```python
from build123d import *

# Parameters (mm, degrees)
SKETCH2_W           = 34
SKETCH2_H           = 27.6
SKETCH2_R           = 2
BOSS_EXTRUDE1_DEPTH = 4
SKETCH3_W           = 34
SKETCH3_H           = 4
BOSS_EXTRUDE2_DEPTH = 47
FILLET1_R           = 9
SKETCH4_R           = 4.5
CUT_EXTRUDE1_DEPTH  = 5


with BuildPart() as part:
    # Sketch2 → Boss-Extrude1 (new body)
    with BuildSketch(Plane(origin=(0, 0, 0), x_dir=(1, 0, 0), z_dir=(0, 1, 0))):
        Rectangle(SKETCH2_W, SKETCH2_H)
        with Locations((0, -7.8)):
            Circle(SKETCH2_R, mode=Mode.SUBTRACT)
    extrude(amount=BOSS_EXTRUDE1_DEPTH)

    # Sketch3 → Boss-Extrude2 (add)
    with BuildSketch(Plane(origin=(0, 4, 0), x_dir=(1, 0, 0), z_dir=(0, 1, 0))):
        with Locations((0, 11.8)):
            Rectangle(SKETCH3_W, SKETCH3_H)
    extrude(amount=BOSS_EXTRUDE2_DEPTH)

    # Fillet1
    fillet1_edges = [part.edges().sort_by_distance(p)[0] for p in [
        (-17, 51, -11.8),
        (17, 51, -11.8),
    ]]
    fillet(fillet1_edges, radius=FILLET1_R)

    # Sketch4 → Cut-Extrude1 (cut, through all)
    with BuildSketch(Plane.XY.offset(-9.8)):
        with Locations((0, 39)):
            Circle(SKETCH4_R)
    extrude(amount=-CUT_EXTRUDE1_DEPTH, mode=Mode.SUBTRACT)


solid = part.part
```
CAD build for the part. Positions are in the model's coordinates, mm. Round coordinates to 2 decimals unless told otherwise and drop trailing zeros. Loops run counter-clockwise (first coordinate to the right, second up) from the corner with the lowest first, then second, coordinate; pieces in that order, holes last. Notation, with made-up numbers: (72, -22.75) - (114, -22.75) arc R21 cw to (114, -2.75) - close; hole circle Ø2 at (-27, 18). An arc over 180 degrees is marked (long way). Return JSON: item names as keys, results as strings. Group by question number.
Q1. Flat gauge pin, fed straight in: pin 1 Ø5 at (x, y) = (11, 42) entering from +Z. Where does the tip first touch, or does it go through?
Q2. Two-plate mould, pull along Y, no slides. Class faces 1 (the face through (0, 27, -9.8)), 2 (the face through (0, 4, 2)), 3 (the face through (-0.98, 34.61, -11.77)): +Y half, -Y half, draft (parallel to the pull), parting line (faces both ways), or undercut.
Q3. Band-saw the part on B-B on z = -11. Give the cut face in (x, y), plus the area to 3 significant figures.
Q4. Band-saw the part on A-A on z = 7.8. Give the cut face in (x, y).
Q5. Drill centre lines: line 1 along X through (y, z) = (1.4, 7.8); line 2 along Z through (x, y) = (0, 2); line 3 along Y through (x, z) = (0, -10.7). Where is each one in solid material? Low to high. Write a range as [from, to].
Q6. Band-saw the part on D-D on x = 0. Give the cut face in (y, z), plus the area to 3 significant figures.
Q7. Band-saw the part on C-C on y = 39. Give the cut face in (x, z).
Solutions:
{
 "1": {"pin 1": "stops at z = -9.8"},
 "2": {"face 1": "draft", "face 2": "+Y half", "face 3": "undercut"},
 "3": {"outline": "(-17, 0) - (17, 0) - (17, 42) arc R9 ccw to (8, 51) - (-8, 51) arc R9 ccw to (-17, 42) - close; hole circle Ø9 at (0, 39)", "area": "1,640 mm^2"},
 "4": {"outline": "(-17, 0) - (-2, 0) - (-2, 4) - (-17, 4) - close; (2, 0) - (17, 0) - (17, 4) - (2, 4) - close"},
 "5": {"line 1": "x = [-17, -2], [2, 17]", "line 2": "z = [-13.8, 5.8], [9.8, 13.8]", "line 3": "y = [0, 34.5], [43.5, 51]"},
 "6": {"outline": "(0, -13.8) - (34.5, -13.8) - (34.5, -9.8) - (4, -9.8) - (4, 5.8) - (0, 5.8) - close; (0, 9.8) - (4, 9.8) - (4, 13.8) - (0, 13.8) - close; (43.5, -13.8) - (51, -13.8) - (51, -9.8) - (43.5, -9.8) - close", "area": "246 mm^2"},
 "7": {"outline": "(-17, -13.8) - (-4.5, -13.8) - (-4.5, -9.8) - (-17, -9.8) - close; (4.5, -13.8) - (17, -13.8) - (17, -9.8) - (4.5, -9.8) - close"}
}
